The figure shows three views and two pictorial views of one solid part (mm, origin at its lowest corner). Answer the questions. Coordinates: 2 decimals unless noted, no trailing zeros. Order: outer loops, then holes, each group sorted by start corner. A loop starts at its lowest first (then second) coordinate and runs counter-clockwise, first axis right, second up. Notation, with made-up numbers: M -21,-24.75 L -13,-24.75 A29 cw -13,-4.75 Z; hole C -1,82 d5. An arc over 180 degrees is marked long. Use a Markdown table: item, result.
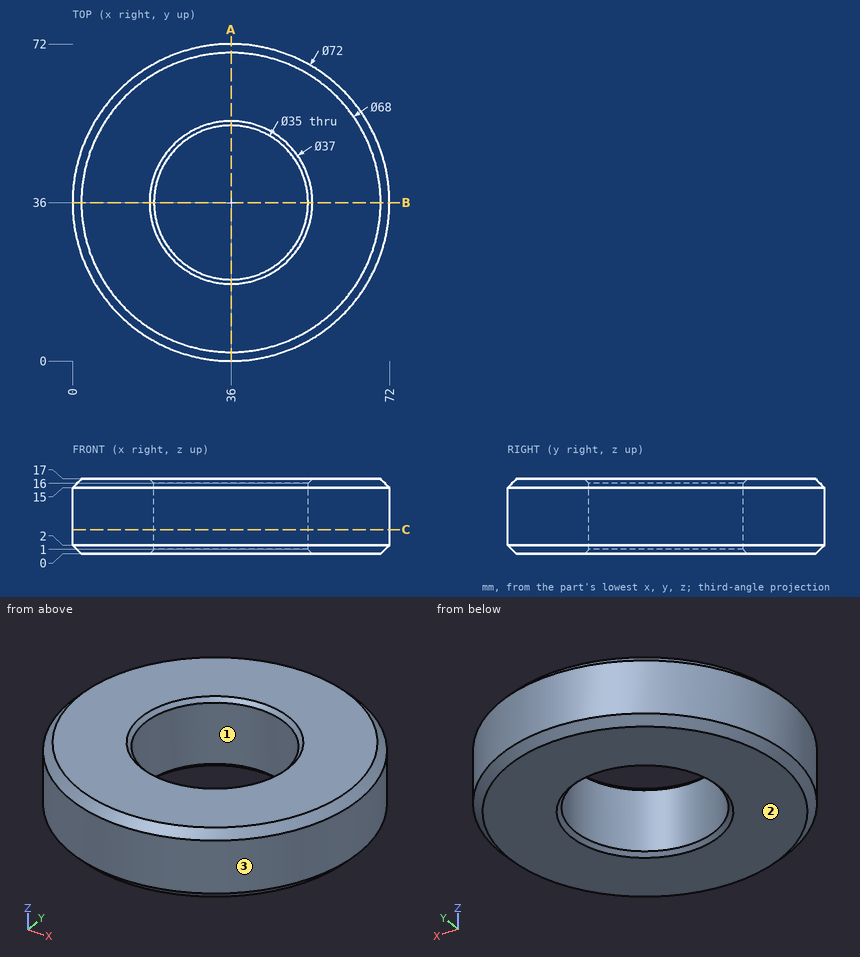
1. Section A-A on x = 36 is taken. Determine the outline of the cut face in (y, z), then the cut area to 3 significant figures.
Answers below:
| item | result |
|---|---|
| outline | M 0,2 L 2,0 L 17.5,0 L 18.5,1 L 18.5,16 L 17.5,17 L 2,17 L 0,15 Z; M 53.5,1 L 54.5,0 L 70,0 L 72,2 L 72,15 L 70,17 L 54.5,17 L 53.5,16 Z |
| area | 619 mm² |
2. For a pull along Y with two mould halves and no side action, classify the marked faces 1, 2 and 3 as +Y half, -Y half, draft (parallel to the pull), parting line (faces both ways), or undercut.
Answers below:
| item | result |
|---|---|
| face 1 | undercut |
| face 2 | draft |
| face 3 | parting line |
3. Section C-C on z = 5.5 is taken. Determine the outline of the cut face in (x, y).
Answers below:
| item | result |
|---|---|
| outline | C 36,36 d72; hole C 36,36 d35 |
4. Flat-ended cylindrical pins translate along their axes: P1, Ø2, axis at y = 12.5, z = 4, coming from the -X side; P2, Ø2, axis at y = 37.5, z = 10.5, coming from the -X side; P3, Ø1, axis at x = 14, z = 13, coming from the +Y side. Find the tip coordinate at first contact, or state that the pin passes through.
Answers below:
| item | result |
|---|---|
| P1 | x = 7.9 |
| P2 | x = 0 |
| P3 | y = 64.87 |
5. Find the intervals of material crossed by probe 1 along Y at (x, z) = (36, 7); probe 2 along X at (y, z) = (23, 7); probe 3 along X at (y, z) = (50.5, 4.75), in increasing order.
Answers below:
| item | result |
|---|---|
| probe 1 | 0 to 18.5, 53.5 to 72 |
| probe 2 | 2.43 to 24.28, 47.72 to 69.57 |
| probe 3 | 3.05 to 26.2, 45.8 to 68.95 |
